Source: three-view drawing plus pictorial views. Frame: mm from the lowest corner of the part. A direction names the side the tool comes from. Give positions to 0.01 mm unless a question says otherwise; leave off trailing zeros. Loops run counter-clockwise (first coordinate to the right, second up) from the corner with the lowest first, then second, coordinate; pieces in that order, holes last. Notation, with made-up numbers: M 83.5,-9 L 141.5,-9 A29 cw 141.5,25 Z; hole C 35,85.5 d2. An arc over 180 degrees is marked long. Write item = value, one per line.
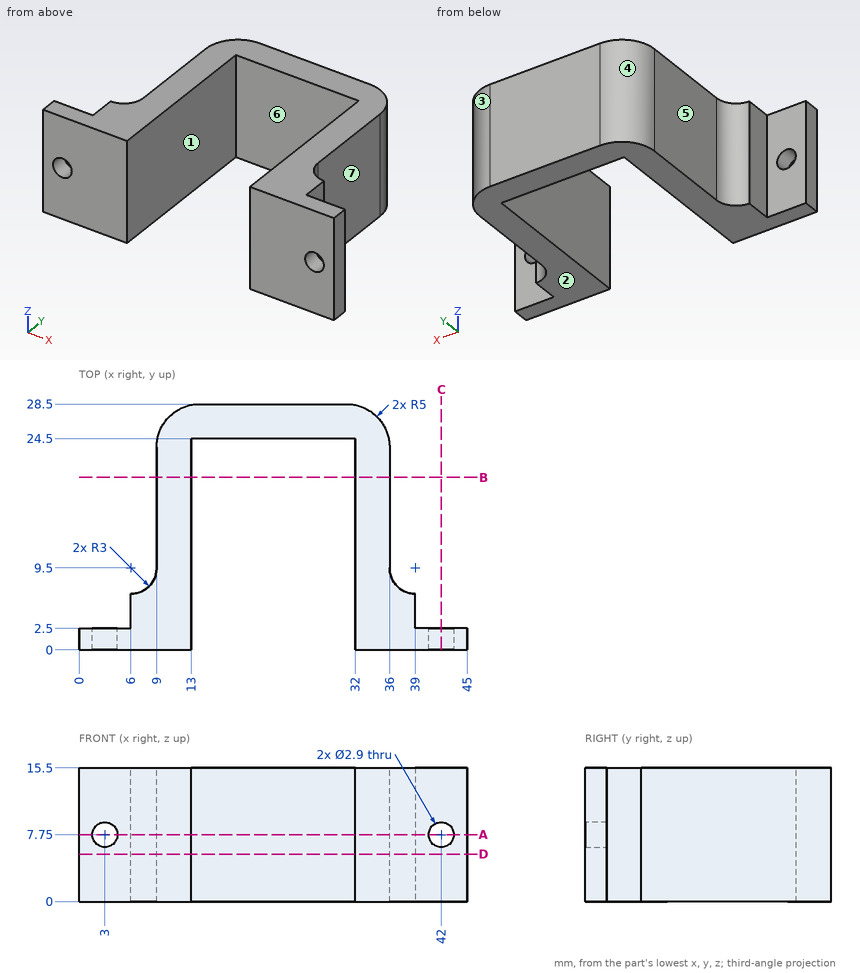
1. First-contact query: pin 1 Ø1 at (x, z) = (21.5, 3) entering from -Y; pin 2 Ø1.8 at (x, z) = (43.5, 11.5) entering from +Y; pin 3 Ø3 at (y, z) = (5, 10.5) entering from -X. Flat tips, straight axial feed; report the tip coordinate or a pass-through.
Derived:
pin_1 = 24.5
pin_2 = 2.5
pin_3 = 6
2. Pull-direction query (X, two-part tool) for the marked faces 1, 2, 3 and 4; classes: +X half, -X half, draft (parallel to the pull), parting line (faces both ways), or undercut.
Derived:
face_1 = undercut
face_2 = draft
face_3 = +X half
face_4 = -X half
3. Material intervals for probe 1 along X at (y, z) = (1.1, 7.75); probe 2 along Z at (x, y) = (42, 1.75); probe 3 along X at (y, z) = (13.5, 8.25), sorted ascending. Write a range as from..to.
Derived:
probe_1 = 0..1.55, 4.45..13, 32..40.55, 43.45..45
probe_2 = 0..6.3, 9.2..15.5
probe_3 = 9..13, 32..36
4. Reachability of the marked faces 5, 6 and 7 from +Z, -Z, +X, -X, +Y, -Y: full face, straight path, thin tool, end or side. Return the list, or none.
Derived:
face_5 = +Z, -Z, -X, +Y
face_6 = +Z, -Z, -Y
face_7 = +Z, -Z, +X, +Y
5. Cut plane C-C, the plane x = 42. Return the cut outline in (y, z).
Derived:
outline = M 0,0 L 2.5,0 L 2.5,6.3 L 0,6.3 Z; M 0,9.2 L 2.5,9.2 L 2.5,15.5 L 0,15.5 Z
6. Cut plane B-B, the plane y = 20. Return the cut outline in (x, z), then the cut area to 3 significant figures.
Derived:
outline = M 9,0 L 13,0 L 13,15.5 L 9,15.5 Z; M 32,0 L 36,0 L 36,15.5 L 32,15.5 Z
area = 124 mm²
7. Cut plane D-D, the plane z = 5.5. Return the cut outline in (x, y), then the cut area to 3 significant figures.
Derived:
outline = M 0,0 L 13,0 L 13,24.5 L 32,24.5 L 32,0 L 45,0 L 45,2.5 L 39,2.5 L 39,6.5 A3 cw 36,9.5 L 36,23.5 A5 ccw 31,28.5 L 14,28.5 A5 ccw 9,23.5 L 9,9.5 A3 cw 6,6.5 L 6,2.5 L 0,2.5 Z
area = 366 mm²
8. Cut plane A-A, the plane z = 7.75. Return the cut outline in (x, y).
Derived:
outline = M 0,0 L 1.55,0 L 1.55,2.5 L 0,2.5 Z; M 4.45,0 L 13,0 L 13,24.5 L 32,24.5 L 32,0 L 40.55,0 L 40.55,2.5 L 39,2.5 L 39,6.5 A3 cw 36,9.5 L 36,23.5 A5 ccw 31,28.5 L 14,28.5 A5 ccw 9,23.5 L 9,9.5 A3 cw 6,6.5 L 6,2.5 L 4.45,2.5 Z; M 43.45,0 L 45,0 L 45,2.5 L 43.45,2.5 Z
